Here's how the part is built. I have some questions about the finished solid (model axes, mm). A direction names the side the tool comes from. Coordinates: 2 decimals unless noted, no trailing zeros. Loops run counter-clockwise (first coordinate to the right, second up) from the corner with the lowest first, then second, coordinate; pieces in that order, holes last. Notation, with made-up numbers: (87, 77.5) -> (129, 77.5) arc R28 cw to (129, 98.5) -> close; hole circle Ø10 at (29, 60). An arc over 180 degrees is marked (long way). Answer as a JSON object with one key per item and string values. Group by question number.
1) I want a section at B-B (z = 3). Write out the boundary of the cut face in (x, y).
2) I want a section at A-A (y = 0). Write out the boundary of the cut face in (x, z).
3) I'm going to push flat-ended pins straight in: pin 1 (1 mm diameter, centred on y = -0.5, z = -2.5, fed in from +X); pin 2 (4 mm diameter, centred on x = 0.5, z = -5.5, fed in from +Y); pin 3 (1.2 mm diameter, centred on x = 0, y = 0.5, fed in from +Z). Where does each tip first touch, or does it pass through?
4) I need wall thicknesses on probe 1 along Z at (x, y) = (1, -2); probe 2 along Y at (x, z) = (0.5, 2); probe 3 along X at (y, z) = (-0.25, 0.5). Which ranges of each line are inside material? Lowest first, please. Write a range as [from, to].
5) If we mould it in two halves opening along X, with no side actions, what happens to faces 4 (the flat face through (0.758, -1.294, 2.763)), 5 (the cylindrical face through (0, 2, -5)), 6 (the flat face through (0, 0, 1.5)), 7 (the flat face through (0, 0, -10))? For each: +X half, -X half, draft (parallel to the pull), parting line (faces both ways), or undercut.
6) Which directions (+Z, -Z, +X, -X, +Y, -Y) give clear straight access to the entire face, cutting with the end or side of a thin tool? Please do faces 1 (the flat face through (2, 0, 4)), 2 (the flat face through (1, -2, 0)), 3 (the cylindrical face through (-0.8, -1.37, 3.91)).
7) I want a section at C-C (z = -7.25). Write out the boundary of the cut face in (x, y).
Autodesk Inventor part; units mm, degrees
ref_plane "YZ Plane" through (0, 0, 0) normal (1, 0, 0) x (0, 1, 0)
ref_plane "XZ Plane" through (0, 0, 0) normal (0, 1, 0) x (-1, 0, 0)
ref_plane "XY Plane" through (0, 0, 0) normal (0, 0, 1) x (1, 0, 0)
sketch "スケッチ1" plane through (0, 0, 0) normal (0, 0, 1) x (1, 0, 0)
  circle A0 centre (0, 0) radius 3.5
  dimension "d0" = 7
extrude "押し出し1" add sketch "スケッチ1" along normal blind 4
sketch "スケッチ2" plane through (0, 0, 0) normal (0, 0, -1) x (-1, 0, 0)
  circle A0 centre (0, 0) radius 3.5
  circle A1 centre (0, 0) radius 2
  dimension "d3" = 4
extrude "押し出し2" add sketch "スケッチ2" along normal blind 10 contours A1
sketch "スケッチ3" plane through (0, 0, 4) normal (0, 0, 1) x (1, 0, 0)
  circle A0 centre (0, 0) radius 3.5
  line L0 (0, 1.7321) -> (1.5, 0.866)
  line L1 (1.5, 0.866) -> (1.5, -0.866)
  line L2 (1.5, -0.866) -> (0, -1.7321)
  line L3 (0, -1.7321) -> (-1.5, -0.866)
  line L4 (-1.5, -0.866) -> (-1.5, 0.866)
  line L5 (-1.5, 0.866) -> (0, 1.7321)
  dimension "d6" = 1.5
extrude "押し出し3" cut sketch "スケッチ3" against normal blind 2.5 contours L0 L1 L2 L3 L4 L5
thread "ねじ1"
fillet "フィレット1" radius 0.5 2 edges at (-3.5, 0, 4) (-3.5, 0, 0)
fillet "フィレット2" radius 0.3 19 edges at (-0.75, 1.299, 4) (-1.5, 0, 4) (-0.75, -1.299, 4) (0.75, -1.299, 4) (1.5, 0, 4) (0.75, 1.299, 4) (-0.75, 1.299, 1.5) (0.75, 1.299, 1.5) (0, 1.7321, 2.75) (-1.5, 0.866, 2.75) (-0.75, -1.299, 1.5) (-1.5, -0.866, 2.75) (-1.5, 0, 1.5) (1.5, 0, 1.5) (1.5, 0.866, 2.75) (1.5, -0.866, 2.75) (0.75, -1.299, 1.5) (0, -1.7321, 2.75) (2, 0, -10)
Determined:
{
 "1": {"outline": "circle Ø7 at (0, 0); hole (-1.5, -0.69) arc R0.3 ccw to (-1.35, -0.95) -> (-0.15, -1.65) arc R0.3 ccw to (0.15, -1.65) -> (1.35, -0.95) arc R0.3 ccw to (1.5, -0.69) -> (1.5, 0.69) arc R0.3 ccw to (1.35, 0.95) -> (0.15, 1.65) arc R0.3 ccw to (-0.15, 1.65) -> (-1.35, 0.95) arc R0.3 ccw to (-1.5, 0.69) -> close"},
 "2": {"outline": "(-3.5, 0.5) arc R0.5 ccw to (-3, 0) -> (-2, 0) -> (-2, -9.7) arc R0.3 ccw to (-1.7, -10) -> (1.7, -10) arc R0.3 ccw to (2, -9.7) -> (2, 0) -> (3, 0) arc R0.5 ccw to (3.5, 0.5) -> (3.5, 3.5) arc R0.5 ccw to (3, 4) -> (1.8, 4) arc R0.3 ccw to (1.5, 3.7) -> (1.5, 1.8) arc R0.3 cw to (1.2, 1.5) -> (-1.2, 1.5) arc R0.3 cw to (-1.5, 1.8) -> (-1.5, 3.7) arc R0.3 ccw to (-1.8, 4) -> (-3, 4) arc R0.5 ccw to (-3.5, 3.5) -> close"},
 "3": {"pin 1": "x = 2", "pin 2": "y = 2", "pin 3": "z = 1.5"},
 "4": {"probe 1": "[0, 4]", "probe 2": "[-3.46, -1.44], [1.44, 3.46]", "probe 3": "[-3.49, 3.49]"},
 "5": {"face 4": "undercut", "face 5": "parting line", "face 6": "undercut", "face 7": "draft"},
 "6": {"face 1": "+Z, +X, -X, +Y, -Y", "face 2": "-Z", "face 3": "+Z"},
 "7": {"outline": "circle Ø4 at (0, 0)"}
}
